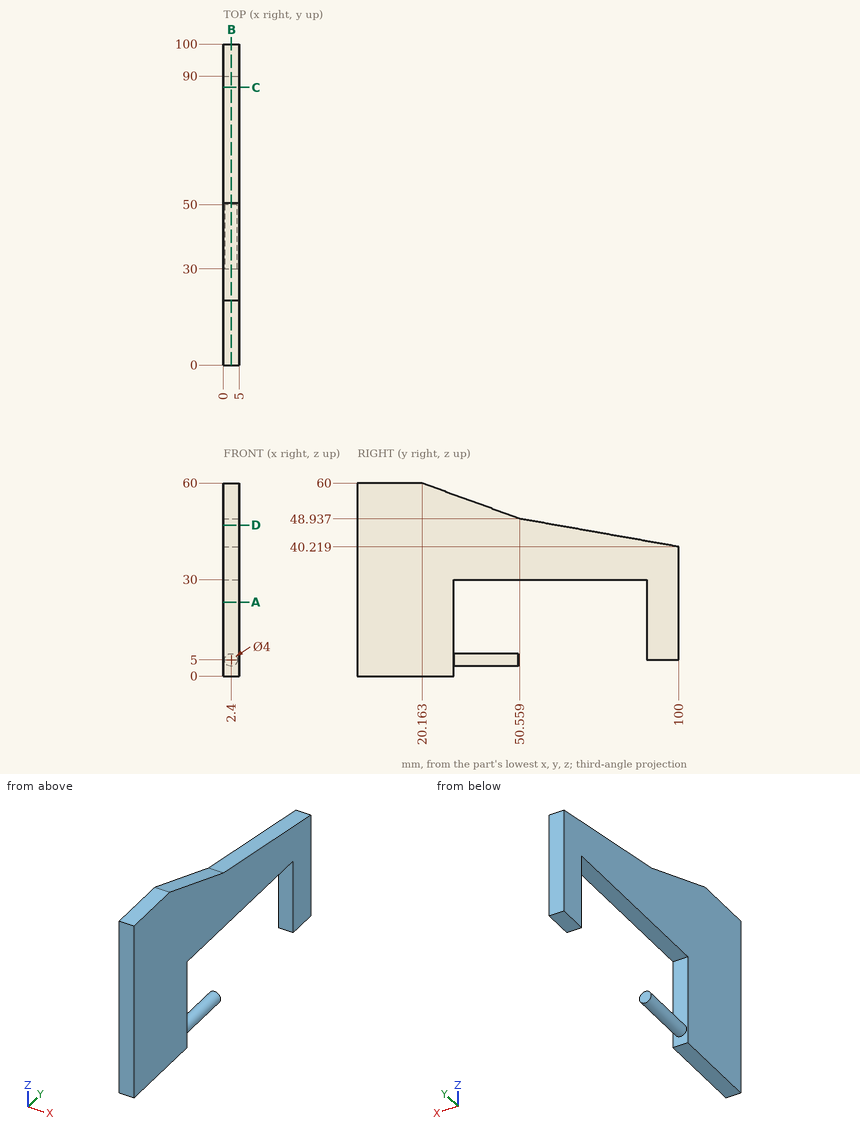
The figure shows three views and two pictorial views of one solid part (mm, origin at its lowest corner). Answer the questions. Give positions to 0.01 mm unless a question says otherwise; leave off trailing zeros. Order: outer loops, then holes, each group sorted by start corner. A loop starts at its lowest first (then second) coordinate and runs counter-clockwise, first axis right, second up. Notation, with made-up numbers: (-6.75, 46) -> (49.25, 46) arc R14 cw to (49.25, 70) -> close; hole circle Ø7 at (65.5, 68). An arc over 180 degrees is marked (long way). Answer as CSV lines item,"result". Start each with the question number.
(1) Section A-A, the plane z = 23 is taken. Write down the section's boundary in (x, y), plus the area to 3 significant figures.
(2) Consider line 1 along Y through (x, z) = (1.5, 15); line 2 along Z through (x, y) = (1.05, 45) (1 decimal); line 3 along Y through (x, z) = (3.6, 4.5). Determine where each line is inside the solid, lowest interval first.
(3) Section C-C, the plane y = 86.5 is taken. Write down the section's boundary in (x, z).
(4) Each of these flat-tipped pins is pushed along its axis until it touches: pin 1 Ø3 at (y, z) = (80, 37.5) entering from -X; pin 2 Ø1.5 at (x, y) = (1.5, 97) entering from -Z. Where does it stop, or does it pass through?
(5) Section D-D, the plane z = 47 is taken. Write down the section's boundary in (x, y).
(6) Section B-B, the plane x = 2.5 is taken. Write down the section's boundary in (y, z).
Entries:
1,outline,"(0, 0) -> (5, 0) -> (5, 30) -> (0, 30) -> close; (0, 90) -> (5, 90) -> (5, 100) -> (0, 100) -> close"
1,area,"200 mm²"
2,line 1,"0 to 30, 90 to 100"
2,line 2,"3.5 to 6.5, 30 to 51"
2,line 3,"0 to 50"
3,outline,"(0, 30) -> (5, 30) -> (5, 42.6) -> (0, 42.6) -> close"
4,pin 1,"x = 0"
4,pin 2,"z = 5"
5,outline,"(0, 0) -> (5, 0) -> (5, 61.54) -> (0, 61.54) -> close"
6,outline,"(0, 0) -> (30, 0) -> (30, 3) -> (50, 3) -> (50, 7) -> (30, 7) -> (30, 30) -> (90, 30) -> (90, 5) -> (100, 5) -> (100, 40.22) -> (50.56, 48.94) -> (20.16, 60) -> (0, 60) -> close"
